Verification items for the finished model (mm, model axes). A direction names the side the tool comes from. Give positions to 0.01 mm unless a question says otherwise; leave off trailing zeros. Loops run counter-clockwise (first coordinate to the right, second up) from the corner with the lowest first, then second, coordinate; pieces in that order, holes last. Notation, with made-up numbers: (-39.5, 47.25) - (0.5, 47.25) arc R14 ccw to (0.5, 66.25) - close; hole circle Ø6 at (-4, 24.25). An arc over 180 degrees is marked (long way). One line per item, written item: value. Start each with the question number.
1. Scan lines: L1, parallel to X at y = 0.75, z = -184 (3 decimals); L2, parallel to Y at x = -3, z = 103 (3 decimals). Record each from-to range of solid material in increasing order. Write a range as [from, to].
2. Gauge pin test, flat ends, axial feed: pin 1 (3 mm diameter, centred on x = -4.5, y = 8.5, fed in from -Z); pin 2 (6 mm diameter, centred on y = 0, z = 50.8, fed in from +X); pin 3 (6.5 mm diameter, centred on y = 0, z = -50.8, fed in from +X). Record the tip position at first contact, or that the pin passes through.
3. Sectioned sample at B-B (z = 70). Record the cut outline in (x, y) (3 decimals).
4. Mould release check, pull along X, two halves, no side actions. Record for faces 3 (the flat face through (0, 9.525, -55)), 4 (the conical face through (16.145, -0.805, 53.358)), 5 (the flat face through (0, 12.7, -5)), 6 (the flat face through (-15.875, 0, -5)): pulls with the +X half, pulls with the -X half, needs draft (parallel to the pull), parting line crosses it, or undercut.
5. Sectioned sample at A-A (x = -1). Record the cut outline in (y, z) (3 decimals).
6. Access from +Z, -Z, +X, -X, +Y, -Y to the whole of each face (thin tool, end or side, straight path). Record for faces 1 (the flat face through (15.875, 0, -5)), 2 (the conical face through (16.145, -0.805, -48.242)).
from build123d import *

# Parameters (mm, degrees)
BOSS_EXTRUDE1_DEPTH             = 330.5556
BOSS_EXTRUDE1_DEPTH_BACK        = 330.5556
SKETCH3_W                       = 38.1
SKETCH3_H                       = 25.4
SKETCH3_W_2                     = 31.75
SKETCH3_H_2                     = 19.05
F_10_CLEARANCE_HOLE2_D          = 5.1054
F_10_0_1935_DIAMETER_HOLE1_D    = 4.9149
F_10_0_1935_DIAMETER_HOLE2_D    = 4.9149
F_10_CLEARANCE_HOLE3_AT_2_COUNT = 2
F_10_CLEARANCE_HOLE3_AT_2_PITCH = 101.6


with BuildPart() as part:
    # Sketch3 → Boss-Extrude1 (new, two sides: drawn at the far end of the back side and taken through both)
    with BuildSketch(Plane.XY.offset(-BOSS_EXTRUDE1_DEPTH_BACK)):
        Rectangle(SKETCH3_W, SKETCH3_H)
        Rectangle(SKETCH3_W_2, SKETCH3_H_2, mode=Mode.SUBTRACT)
    extrude(amount=BOSS_EXTRUDE1_DEPTH + BOSS_EXTRUDE1_DEPTH_BACK)

    # #10 Clearance Hole2 (through all)
    with Locations(Plane.ZY.offset(19.05)):
        with Locations((-317.8556, 0), (-292.4556, 0), (292.4556, 0), (317.8556, 0)):
            Hole(F_10_CLEARANCE_HOLE2_D / 2)

    # #10 (0.1935) Diameter Hole1 (through all)
    with Locations(Plane(origin=(19.05, 0, 0), x_dir=(0, 0, -1), z_dir=(1, 0, 0))):
        with Locations((-261.128868491, 0.3559048), (-235.728868491, 0.3559048), (-230.046541854, 8.473619523), (-132.984885112, 1.9434048), (-107.584885112, 1.9434048)):
            Hole(F_10_0_1935_DIAMETER_HOLE1_D / 2)

    # #10 (0.1935) Diameter Hole2 (through all)
    with Locations(Plane(origin=(19.05, 0, 0), x_dir=(0, 0, -1), z_dir=(1, 0, 0))):
        with Locations((-261.840668479, 0), (-236.440668479, 0)):
            Hole(F_10_0_1935_DIAMETER_HOLE2_D / 2)

    # Sketch21 → #10 Clearance Hole3 (revolve, cut)
    with BuildSketch(Plane(origin=(-19.05, 0, -50.8), x_dir=(0, 0, 1), z_dir=(0, 1, 0))):
        Polygon((0, 0), (0, 38.1), (5.207, 38.1), (2.5527, 35.046577137), (2.5527, 0), align=None)
    f_10_clearance_hole3 = revolve(axis=Axis((-25.4, 0, -50.8), (1, 0, 0)), mode=Mode.SUBTRACT)

    # #10 Clearance Hole3 at 2: #10 Clearance Hole3 ×2
    with Locations(*[(0, 0, i * F_10_CLEARANCE_HOLE3_AT_2_PITCH) for i in range(1, F_10_CLEARANCE_HOLE3_AT_2_COUNT)]):
        add(f_10_clearance_hole3, mode=Mode.SUBTRACT)


solid = part.part
Results are:
1. L1: x = [-19.05, -15.875], [15.875, 19.05]
1. L2: y = [-12.7, -9.525], [9.525, 12.7]
2. pin 1: stops at z = -330.56
2. pin 2: stops at x = 16.51
2. pin 3: stops at x = 16.8
3. outline: (-19.05, -12.7) - (19.05, -12.7) - (19.05, 12.7) - (-19.05, 12.7) - close; hole (-15.875, -9.525) - (15.875, -9.525) - (15.875, 9.525) - (-15.875, 9.525) - close
4. face 3: undercut
4. face 4: pulls with the +X half
4. face 5: needs draft
4. face 6: undercut
5. outline: (-12.7, -330.556) - (-9.525, -330.556) - (-9.525, 330.556) - (-12.7, 330.556) - close; (9.525, -330.556) - (12.7, -330.556) - (12.7, 330.556) - (9.525, 330.556) - (9.525, 232.268) arc R2.457 cw to (9.525, 227.825) - close
6. face 1: +Z, -Z
6. face 2: +X
